CAD build for the part. Positions are in the model's coordinates, mm. A direction names the side the tool comes from. Round coordinates to 2 decimals unless told otherwise and drop trailing zeros. Loops run counter-clockwise (first coordinate to the right, second up) from the corner with the lowest first, then second, coordinate; pieces in that order, holes last. Notation, with made-up numbers: M 11,82 L 34,82 A15 ccw 34,87 Z; hole C 48,13.5 d1. An arc over 180 degrees is marked long. Put each result on its own line as item: value. Start each with the question number.
from build123d import *

# Parameters (mm, degrees)
FASE1_SIZE                            = 1.6
SCHNITT_LINEAR_AUSTRAGEN1_DEPTH       = 24
F_5_5_5_5_DURCHMESSER_BOHRUNG1_D      = 5.5
M4_GEWINDEBOHRUNG2_D                  = 3.3
M4_GEWINDEBOHRUNG2_DEPTH              = 22
M4_GEWINDEBOHRUNG2_TIP                = 0.991420021
F_0_8_0_8_DURCHMESSER_BOHRUNG1_REACH  = 55.819
F_0_8_0_8_DURCHMESSER_BOHRUNG1_BORE_R = 0.4
KREISMUSTER1_COUNT                    = 3


with BuildPart() as part:
    # Skizze1 → Rotation1 (revolve)
    with BuildSketch(Plane.XY):
        Polygon((21.5, 0), (32.5, 0), (32.5, 15.51125461), (20, 26), (20, 28), (14.25, 28), (14.25, 18.75), (21.5, 11.5), align=None)
    revolve(axis=Axis((0, 0, 0), (0, 1, 0)))

    # Fase1
    fase1_edges = [part.edges().sort_by_distance(p)[0] for p in [
        (-21.5, 0, 0),
    ]]
    chamfer(fase1_edges, length=FASE1_SIZE)

    # Skizze2 → Schnitt-Linear austragen1 (cut)
    with BuildSketch(Plane(origin=(0, 28, 0), x_dir=(1, 0, 0), z_dir=(0, 1, 0))):
        with BuildLine():
            Line((27.5, 5), (36.713219287, 5))
            ThreePointArc((36.713219287, 5), (41.713219287, 0), (36.713219287, -5))
            Line((36.713219287, -5), (27.5, -5))
            ThreePointArc((27.5, -5), (22.5, 0), (27.5, 5))
        make_face()
    extrude(amount=-SCHNITT_LINEAR_AUSTRAGEN1_DEPTH, mode=Mode.SUBTRACT)

    # 5.5 _5.5_ Durchmesser Bohrung1 (through all)
    with Locations(Plane(origin=(0, 28, 0), x_dir=(1, 0, 0), z_dir=(0, 1, 0))):
        with Locations((27.5, 0)):
            Hole(F_5_5_5_5_DURCHMESSER_BOHRUNG1_D / 2)

    # Skizze9 → Schnitt-Rotation1 (revolve, cut)
    with BuildSketch(Plane.XY):
        Polygon((-34.391087084, 3.108912916), (-31.792893219, 5.707106781), (-30.201902961, 4.116116524), (-32.800096827, 1.517922658), align=None)
    revolve(axis=Axis((-34.391087084, 3.108912916, 0), (0.7071067811865462, 0.7071067811865488, 0)), mode=Mode.SUBTRACT)

    # M4 Gewindebohrung2
    with Locations(Plane(origin=(-13.042893219, -13.042893219, 0), x_dir=(-0.7071067811865488, 0.7071067811865462, 0), z_dir=(-0.7071067811865462, -0.7071067811865488, 0))):
        with Locations((26.516504294, 0)):
            Hole(M4_GEWINDEBOHRUNG2_D / 2, depth=M4_GEWINDEBOHRUNG2_DEPTH)
            with Locations((0, 0, -(M4_GEWINDEBOHRUNG2_DEPTH + M4_GEWINDEBOHRUNG2_TIP / 2))):  # 118° drill point
                Cone(0, M4_GEWINDEBOHRUNG2_D / 2, M4_GEWINDEBOHRUNG2_TIP, mode=Mode.SUBTRACT)

    # 0.8 _0.8_ Durchmesser Bohrung1 bore → 0.8 _0.8_ Durchmesser Bohrung1 (cut, up to next)
    with BuildSketch(Plane(origin=(0, 28, 0), x_dir=(1, 0, 0), z_dir=(0, 1, 0)), mode=Mode.PRIVATE) as f_0_8_0_8_durchmesser_bohrung1_sk1:
        with Locations((-15.875, 0)):
            Circle(F_0_8_0_8_DURCHMESSER_BOHRUNG1_BORE_R)
    f_0_8_0_8_durchmesser_bohrung1_tool1 = extrude(f_0_8_0_8_durchmesser_bohrung1_sk1.sketch, amount=-F_0_8_0_8_DURCHMESSER_BOHRUNG1_REACH, mode=Mode.PRIVATE) & part.part
    f_0_8_0_8_durchmesser_bohrung1 = f_0_8_0_8_durchmesser_bohrung1_tool1.solids().sort_by_distance((-15.875, 28, 0))[0]
    add(f_0_8_0_8_durchmesser_bohrung1, mode=Mode.SUBTRACT)

    # Kreismuster1: 0.8 _0.8_ Durchmesser Bohrung1; each copy of 0.8 _0.8_ Durchmesser Bohrung1 runs up to whatever stops it at its own place
    kreismuster1_before = part.part  # the part as the pattern finds it: every copy runs up to it
    kreismuster1_f_0_8_0_8_durchmesser_bohrung1_long = extrude(f_0_8_0_8_durchmesser_bohrung1_sk1.sketch, amount=-F_0_8_0_8_DURCHMESSER_BOHRUNG1_REACH, mode=Mode.PRIVATE)
    kreismuster1_f_0_8_0_8_durchmesser_bohrung1_tool = kreismuster1_f_0_8_0_8_durchmesser_bohrung1_long.rotate(Axis((0, 0, 0), (0, 1, 0)), 1 * 360 / KREISMUSTER1_COUNT) & kreismuster1_before
    add(kreismuster1_f_0_8_0_8_durchmesser_bohrung1_tool.solids().sort_by_distance((7.9375, 28, 13.748153))[0], mode=Mode.SUBTRACT)
    kreismuster1_f_0_8_0_8_durchmesser_bohrung1_tool = kreismuster1_f_0_8_0_8_durchmesser_bohrung1_long.rotate(Axis((0, 0, 0), (0, 1, 0)), 2 * 360 / KREISMUSTER1_COUNT) & kreismuster1_before
    add(kreismuster1_f_0_8_0_8_durchmesser_bohrung1_tool.solids().sort_by_distance((7.9375, 28, -13.748153))[0], mode=Mode.SUBTRACT)

    # Skizze15 → Schnitt-Rotation2 (revolve, cut)
    with BuildSketch(Plane(origin=(-2.039898254, 0, -12.060602687), x_dir=(0, 1, 0), z_dir=(0.16676874671610264, 0, 0.9859960370705049))):
        Polygon((3.231062719, -32.218445859), (5.64278761, -29.344264057), (7.366387607, -30.790536178), (4.954662716, -33.664717981), align=None)
    revolve(axis=Axis((29.727361684, 3.231062719, -17.433632524), (-0.7553167851351978, 0.6427876096865349, 0.12775227170778738)), mode=Mode.SUBTRACT)


solid = part.part
(1) Cut at A-A on x = 0. List the corners of the cut face in (y, z), and give its area (3 significant figures).
(2) Cut at B-B on y = 10. Count the separate pieces of the cut face and the enclosed holes in it, and give its area (3 significant figures).
(3) Mould opens along X. For faces 6 (the cylindrical face through (31, 7.86, -9.76)), 7 (the cylindrical face through (-2.799, 6.481, -21.317)), 8 (the flat face through (-5, 28, -14)) say: +X half, -X half, draft (parallel to the pull), parting line (faces both ways), or undercut.
(4) Drill centre lines: line 1 along Z through (x, y) = (0, 5); line 2 along X through (y, z) = (22, -1); line 3 along Z through (x, y) = (23.5, 17). Where is each one in solid material? Low to high.
(5) Tool access for faces 1 (the conical face through (-15.405, 21.44, -0.02)), 2 (the flat face through (30, 10, 5)), 3 (the cylindrical face through (-4.336, 27.014, 19.524)), 4 (the flat face through (8, 0, -22)), 5 (the cylindrical face through (30.247, 1.972, -0.121)): list every direction of +Z, -Z, +X, -X, +Y, -Y with a clear straight run to the whole face (end or side of a thin tool).
(6) Flat gauge pins, fed straight in: pin 1 Ø1 at (x, z) = (-9.5, 9.5) entering from -Y; pin 2 Ø3 at (y, z) = (6.5, -20.5) entering from +X; pin 3 Ø3 at (y, z) = (18, 10.5) entering from +X; pin 4 Ø5 at (x, z) = (-19.5, -26) entering from -Y. Where does each tip first touch, or does it go through?
Taken from the geometry:
1. outline: M 0,-32.5 L 15.51,-32.5 L 26,-20 L 28,-20 L 28,-14.25 L 18.75,-14.25 L 11.5,-21.5 L 1.6,-21.5 L 0,-23.1 Z; M 0,23.1 L 1.6,21.5 L 11.5,21.5 L 18.75,14.25 L 28,14.25 L 28,20 L 26,20 L 15.51,32.5 L 0,32.5 Z
1. area: 619 mm2
2. separate pieces: 1
2. enclosed holes: 2
2. area: 1,770 mm2
3. face 6: parting line
3. face 7: undercut
3. face 8: draft
4. line 1: -32.5 to -21.5, 21.5 to 32.5
4. line 2: -24.75 to -17.36, -16.68 to -14.21, 14.21 to 22.6
4. line 3: -19.79 to -3, 3 to 19.79
5. face 1: none
5. face 2: +X, +Y
5. face 3: +Y
5. face 4: +Z, -Z, +X, -X, -Y
5. face 5: +Y, -Y
6. pin 1: through
6. pin 2: x = 26.37
6. pin 3: x = 29.58
6. pin 4: y = 0
